Design review of the part built by this model. Coordinates are the model's own, in mm. Face numbers are marked on the shaded views. A direction names the side the tool comes from. Give positions to 0.01 mm unless a question says otherwise; leave off trailing zeros. Write each loop counter-clockwise with the first axis right and the second up, starting at its lowest first coordinate (ties: lowest second). Pieces come first, ordered by that corner, then holes. Notation, with made-up numbers: M 58,16 L 67,16 A16 ccw 67,42 Z; hole C 49,-40 d2. An arc over 180 degrees is marked long. Answer in a Markdown table with one row per item.
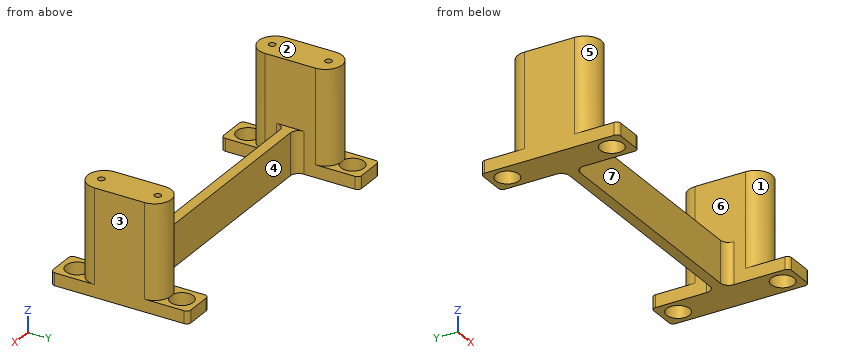
Autodesk Inventor part; units mm, degrees
ref_plane "YZ Plane" through (0, 0, 0) normal (1, 0, 0) x (0, 1, 0)
ref_plane "XZ Plane" through (0, 0, 0) normal (0, 1, 0) x (-1, 0, 0)
ref_plane "XY Plane" through (0, 0, 0) normal (0, 0, 1) x (1, 0, 0)
sketch "Esquisse1" plane through (0, 0, 0) normal (0, 0, 1) x (1, 0, 0)
  line L0 (75, 0) -> (75, 33)
  line L1 (0, 33) -> (0, 0)
  line L2 (8, 33) -> (8, 0)
  line L3 (67, 33) -> (67, 0)
  line L4 (8, 17.75) -> (67, 17.75)
  line L5 (67, 17.75) -> (67, 15.25)
  line L6 (67, 15.25) -> (8, 15.25)
  line L7 (8, 15.25) -> (8, 17.75)
  line L8 (75, 33) -> (67, 33)
  line L9 (8, 33) -> (0, 33)
  line L10 (0, 0) -> (8, 0)
  line L11 (67, 0) -> (75, 0)
  line L12 (1.5, 6.5) -> (6.5, 6.5)
  line L13 (6.5, 6.5) -> (6.5, 1.5)
  line L14 (6.5, 1.5) -> (1.5, 1.5)
  line L15 (1.5, 1.5) -> (1.5, 6.5)
  line L16 (0, 16.5) -> (-2.6312, 16.5)
  line L17 (37.5, 15.25) -> (37.5, 13.3261)
  line L18 (1.5, 26.5) -> (6.5, 26.5)
  line L19 (6.5, 26.5) -> (6.5, 31.5)
  line L20 (6.5, 31.5) -> (1.5, 31.5)
  line L21 (1.5, 31.5) -> (1.5, 26.5)
  line L22 (73.5, 6.5) -> (68.5, 6.5)
  line L23 (68.5, 6.5) -> (68.5, 1.5)
  line L24 (68.5, 1.5) -> (73.5, 1.5)
  line L25 (73.5, 1.5) -> (73.5, 6.5)
  line L26 (68.5, 26.5) -> (68.5, 31.5)
  line L27 (68.5, 31.5) -> (73.5, 31.5)
  line L28 (73.5, 31.5) -> (73.5, 26.5)
  line L29 (73.5, 26.5) -> (68.5, 26.5)
  arc A0 (8, 22.5) -> (0, 22.5) centre (4, 22.5) ccw
  arc A1 (0, 10.5) -> (8, 10.5) centre (4, 10.5) ccw
  arc A2 (75, 22.5) -> (67, 22.5) centre (71, 22.5) ccw
  arc A3 (67, 10.5) -> (75, 10.5) centre (71, 10.5) ccw
  line L30 (67, 22.5) -> (67, 10.5)
  line L31 (75, 10.5) -> (75, 22.5)
  line L32 (8, 22.5) -> (8, 10.5)
  line L33 (0, 10.5) -> (0, 22.5)
  dimension "d0" = 33
  dimension "d1" = 75
  dimension "d2" = 8
  dimension "d3" = 8
  dimension "d4" = 2.5
  dimension "d6" = 5
  dimension "d7" = 5
  dimension "d8" = 1.5
  dimension "d9" = 1.5
  dimension "d10" = 8
  dimension "d11" = 8
  dimension "d12" = 12
  dimension "d13" = 10.5
extrude "Extrusion1" add sketch "Esquisse1" along normal blind 3 contours L11 L3 A3 L0 | A2 L3 L8 L0 | A0 L1 L9 L2 | L2 L10 L1 A1
extrude "Extrusion2" add sketch "Esquisse1" along normal blind 25.5 contours A3 L3 A2 L0 | L2 A1 L1 A0
extrude "Extrusion3" add sketch "Esquisse1" along normal blind 10 contours L6 L2 L4 L3
fillet "Congé1" radius 2 4 edges at (8, 15.25, 5) (8, 17.75, 5) (67, 15.25, 5) (67, 17.75, 5)
hole "Perçage1" at (71, 23.25, 25.5) direction (0, 0, -1) diameter 1.6 depth 10 tip angle 118
hole "Perçage2" at (71, 9.75, 25.5) direction (0, 0, -1) diameter 1.6 depth 10 tip angle 118
hole "Perçage3" at (4, 23.25, 25.5) direction (0, 0, -1) diameter 1.6 depth 10 tip angle 118
hole "Perçage4" at (4, 9.75, 25.5) direction (0, 0, -1) diameter 1.6 depth 10 tip angle 118
fillet "Congé2" radius 1 8 edges at (8, 0, 1.5) (0, 0, 1.5) (67, 0, 1.5) (75, 0, 1.5) (67, 33, 1.5) (75, 33, 1.5) (8, 33, 1.5) (0, 33, 1.5)
sketch "Esquisse3" plane through (0, 0, 3) normal (0, 0, 1) x (1, 0, 0)
  arc A0 (1, 33) -> (0, 32) centre (1, 32) ccw
  line L0 (0, 32) -> (0, 22.5)
  arc A1 (4, 26.5) -> (0, 22.5) centre (4, 22.5) ccw
  line L1 (4, 26.5) -> (1.5, 26.5)
  line L2 (1.5, 26.5) -> (1.5, 31.5)
  line L3 (1.5, 31.5) -> (6.5, 31.5)
  line L4 (6.5, 31.5) -> (6.5, 26.5)
  line L5 (6.5, 26.5) -> (4, 26.5)
  arc A2 (8, 22.5) -> (4, 26.5) centre (4, 22.5) ccw
  line L6 (8, 22.5) -> (8, 32)
  arc A3 (8, 32) -> (7, 33) centre (7, 32) ccw
  line L7 (7, 33) -> (1, 33)
  arc A4 (75, 32) -> (74, 33) centre (74, 32) ccw
  line L8 (74, 33) -> (68, 33)
  arc A5 (68, 33) -> (67, 32) centre (68, 32) ccw
  line L9 (67, 32) -> (67, 22.5)
  arc A6 (71, 26.5) -> (67, 22.5) centre (71, 22.5) ccw
  line L10 (71, 26.5) -> (68.5, 26.5)
  line L11 (68.5, 26.5) -> (68.5, 31.5)
  line L12 (68.5, 31.5) -> (73.5, 31.5)
  line L13 (73.5, 31.5) -> (73.5, 26.5)
  line L14 (73.5, 26.5) -> (71, 26.5)
  arc A7 (75, 22.5) -> (71, 26.5) centre (71, 22.5) ccw
  line L15 (75, 22.5) -> (75, 32)
  arc A8 (74, 0) -> (75, 1) centre (74, 1) ccw
  line L16 (75, 1) -> (75, 10.5)
  arc A9 (71, 6.5) -> (75, 10.5) centre (71, 10.5) ccw
  line L17 (71, 6.5) -> (73.5, 6.5)
  line L18 (73.5, 6.5) -> (73.5, 1.5)
  line L19 (73.5, 1.5) -> (68.5, 1.5)
  line L20 (68.5, 1.5) -> (68.5, 6.5)
  line L21 (68.5, 6.5) -> (71, 6.5)
  arc A10 (67, 10.5) -> (71, 6.5) centre (71, 10.5) ccw
  line L22 (67, 10.5) -> (67, 1)
  arc A11 (67, 1) -> (68, 0) centre (68, 1) ccw
  line L23 (68, 0) -> (74, 0)
  arc A12 (0, 1) -> (1, 0) centre (1, 1) ccw
  line L24 (1, 0) -> (7, 0)
  arc A13 (7, 0) -> (8, 1) centre (7, 1) ccw
  line L25 (8, 1) -> (8, 10.5)
  arc A14 (4, 6.5) -> (8, 10.5) centre (4, 10.5) ccw
  line L26 (4, 6.5) -> (6.5, 6.5)
  line L27 (6.5, 6.5) -> (6.5, 1.5)
  line L28 (6.5, 1.5) -> (1.5, 1.5)
  line L29 (1.5, 1.5) -> (1.5, 6.5)
  line L30 (1.5, 6.5) -> (4, 6.5)
  arc A15 (0, 10.5) -> (4, 6.5) centre (4, 10.5) ccw
  line L31 (0, 10.5) -> (0, 1)
  circle A16 centre (4, 29) radius 2.5
  circle A17 centre (4, 4) radius 2.5
  circle A18 centre (71, 4) radius 2.5
  circle A19 centre (71, 29) radius 2.5
  point P0 (0, 0)
extrude "Extrusion4" add sketch "Esquisse3" against normal up to surface (3 mm away) contours L1 L2 A16 | A16 L4 L5 | A16 L3 L4 | L2 L3 A16 | L10 L11 A19 | A19 L13 L14 | L15 A7 A6 L9 A5 L8 A4 | A19 L12 L13 | L11 L12 A19 | L17 L18 A18 | A18 L20 L21 | L18 L19 A18 | A18 L19 L20 | L26 L27 A17 | A17 L29 L30 | L31 A15 A14 L25 A13 L24 A12 | L27 L28 A17 | A17 L28 L29
sketch "Esquisse4" plane through (0, 0, 0) normal (0, 0, -1) x (-1, 0, 0)
  circle A0 centre (-4, 29) radius 2.5
  circle A1 centre (-4, 4) radius 2.5
  circle A2 centre (-71, 4) radius 2.5
  circle A3 centre (-71, 29) radius 2.5
  circle A4 centre (-4, 29) radius 2.75
  circle A5 centre (-4, 4) radius 2.75
  circle A6 centre (-71, 29) radius 2.75
  circle A7 centre (-71, 4) radius 2.75
  point P0 (0, 0)
  dimension "d61" = 5.5
  dimension "d62" = 5.5
  dimension "d63" = 5.5
  dimension "d64" = 5.5
extrude "Extrusion5" cut sketch "Esquisse4" against normal blind 3
equation "\"d9\" = -0.5 * d6 + 0.5 * d2"
equation "\"d13\" = -0.5 * d12 + 0.5 * d0"
properties part number "red_part-july21" material "Plastique ABS"
1) The part is to be moulded in two halves that separate along X. For the marked faces 1, 2 and 3, say which applies: released by +X, released by -X, zero draft, split by the parting line, or undercut.
Geometry says:
| item | result |
|---|---|
| face 1 | undercut |
| face 2 | zero draft |
| face 3 | released by +X |
2) Add section C-C (y = 25.5). Write out the cut boundary in (x, z).
Geometry says:
| item | result |
|---|---|
| outline | M 0,0 L 8,0 L 8,3 L 6.65,3 L 6.65,25.5 L 1.35,25.5 L 1.35,3 L 0,3 Z; M 67,0 L 75,0 L 75,3 L 73.65,3 L 73.65,25.5 L 68.35,25.5 L 68.35,3 L 67,3 Z |
3) Add section A-A (z = 21). Write out the cut boundary in (x, y), and give its area (3 significant figures).
Geometry says:
| item | result |
|---|---|
| outline | M 0,10.5 A4 ccw 8,10.5 L 8,22.5 A4 ccw 0,22.5 Z; M 67,10.5 A4 ccw 75,10.5 L 75,22.5 A4 ccw 67,22.5 Z; hole C 4,9.75 d1.6; hole C 4,23.25 d1.6; hole C 71,9.75 d1.6; hole C 71,23.25 d1.6 |
| area | 284 mm^2 |
4) To check wall thickness, follow probe 1 along X at (y, z) = (4, 0.9); probe 2 along Y at (x, z) = (71, 1.1); probe 3 along X at (y, z) = (19, 14). State the ranges of each line that lie inside material, in increasing order. Write a range as [from, to].
Geometry says:
| item | result |
|---|---|
| probe 1 | [0, 1.25], [6.75, 8], [67, 68.25], [73.75, 75] |
| probe 2 | [0, 1.25], [6.75, 26.25], [31.75, 33] |
| probe 3 | [0, 8], [67, 75] |
5) Insertion check: P1, Ø6, axis at x = 57, z = 3, coming from the +Y side; P2, Ø6.5, axis at x = 69, y = 3.5, coming from the +Z side; P3, Ø1.3, axis at x = 71, y = 9.75, coming from the +Z side; P4, Ø4.5, axis at x = 4, y = 4, coming from the -Z side. Each pin has a flat end and moves straight along its axis. Give the tip position at first contact, or say it passes through.
Geometry says:
| item | result |
|---|---|
| P1 | y = 17.75 |
| P2 | z = 3 |
| P3 | z = 15.41 |
| P4 | through |
6) Add section D-D (z = 4.75). Write out the cut boundary in (x, y), and give its area (3 significant figures).
Geometry says:
| item | result |
|---|---|
| outline | M 0,10.5 A4 ccw 8,10.5 L 8,13.25 A2 cw 10,15.25 L 65,15.25 A2 cw 67,13.25 L 67,10.5 A4 ccw 75,10.5 L 75,22.5 A4 ccw 67,22.5 L 67,19.75 A2 cw 65,17.75 L 10,17.75 A2 cw 8,19.75 L 8,22.5 A4 ccw 0,22.5 Z |
| area | 443 mm^2 |
7) For the marked faces 4, 5, 6 and 7, list the 3-axis set-ups (+Z, -Z, +X, -X, +Y, -Y) from which the entire face can be reached by the end or side of a thin tool; tool diameter is ignored.
Geometry says:
| item | result |
|---|---|
| face 4 | +Z, -Z, +Y |
| face 5 | +Z, -Y |
| face 6 | +Z |
| face 7 | +Z, -Z, -Y |
8) Add section B-B (y = 29). Write out the cut boundary in (x, z), and give its area (3 significant figures).
Geometry says:
| item | result |
|---|---|
| outline | M 0,0 L 1.25,0 L 1.25,3 L 0,3 Z; M 6.75,0 L 8,0 L 8,3 L 6.75,3 Z; M 67,0 L 68.25,0 L 68.25,3 L 67,3 Z; M 73.75,0 L 75,0 L 75,3 L 73.75,3 Z |
| area | 15.0 mm^2 |
